```python
from build123d import *

# Parameters (mm, degrees)
SKETCH009_R     = 1.6
PAD003_DEPTH    = 2.5
SKETCH010_R     = 1.6
PAD004_DEPTH    = 2.5
FILLET002_R     = 2
SKETCH011_R     = 6.5
SKETCH011_R_2   = 1.6
PAD005_DEPTH    = 2
SKETCH012_R     = 3.2
SKETCH012_R_2   = 1.6
PAD006_DEPTH    = 4.25
FILLET003_R     = 1
POCKET006_DEPTH = 2.5


with BuildPart() as part:
    # Sketch009 → Pad003 (new body)
    with BuildSketch(Plane.XY):
        with BuildLine():
            ThreePointArc((23.646194, 14.453806), (23.646194, 23.646194), (14.453806, 23.646194))
            Line((14.453806, 23.646194), (0, 9.192388))
            Line((-14.453806, 23.646194), (0, 9.192388))
            ThreePointArc((-14.453806, 23.646194), (-23.646194, 23.646194), (-23.646194, 14.453806))
            Line((-9.192388, 0), (-23.646194, 14.453806))
            Line((-23.646194, -14.453806), (-9.192388, 0))
            ThreePointArc((-23.646194, -14.453806), (-23.646194, -23.646194), (-14.453806, -23.646194))
            Line((-14.453806, -23.646194), (0, -9.192388))
            Line((14.453806, -23.646194), (0, -9.192388))
            ThreePointArc((14.453806, -23.646194), (23.646194, -23.646194), (23.646194, -14.453806))
            Line((23.646194, -14.453806), (9.192388, 0))
            Line((23.646194, 14.453806), (9.192388, 0))
        make_face()
        with Locations((19.05, 19.05)):
            Circle(SKETCH009_R, mode=Mode.SUBTRACT)
        with Locations((-19.05, 19.05)):
            Circle(SKETCH009_R, mode=Mode.SUBTRACT)
        with Locations((-19.05, -19.05)):
            Circle(SKETCH009_R, mode=Mode.SUBTRACT)
        with Locations((19.05, -19.05)):
            Circle(SKETCH009_R, mode=Mode.SUBTRACT)
    extrude(amount=PAD003_DEPTH)

    # Sketch010 → Pad004 (join)
    with BuildSketch(Plane.XY):
        with BuildLine():
            ThreePointArc((-25, 4.8), (-29.8, 0), (-25, -4.8))
            Line((-25, -4.8), (25, -4.8))
            ThreePointArc((25, -4.8), (29.8, 0), (25, 4.8))
            Line((25, 4.8), (-25, 4.8))
        make_face()
        with Locations((-25, 0)):
            Circle(SKETCH010_R, mode=Mode.SUBTRACT)
        with Locations((25, 0)):
            Circle(SKETCH010_R, mode=Mode.SUBTRACT)
    extrude(amount=PAD004_DEPTH)

    # Fillet002
    fillet002_edges = [part.edges().sort_by_distance(p)[0] for p in [
        (13.992388, 4.8, 1.25),
        (13.992388, -4.8, 1.25),
        (0, -9.192388, 1.25),
        (-13.992388, -4.8, 1.25),
        (-13.992388, 4.8, 1.25),
        (0, 9.192388, 1.25),
    ]]
    fillet(fillet002_edges, radius=FILLET002_R)

    # Sketch011 (on Face16 of Fillet002) → Pad005 (join)
    with BuildSketch(Plane.XY.offset(2.5)):
        with Locations((-19.05, 19.05)):
            Circle(SKETCH011_R)
        with Locations((-19.05, 19.05)):
            Circle(SKETCH011_R_2, mode=Mode.SUBTRACT)
        with Locations((19.05, 19.05)):
            Circle(SKETCH011_R)
        with Locations((19.05, 19.05)):
            Circle(SKETCH011_R_2, mode=Mode.SUBTRACT)
        with Locations((19.05, -19.05)):
            Circle(SKETCH011_R)
        with Locations((19.05, -19.05)):
            Circle(SKETCH011_R_2, mode=Mode.SUBTRACT)
        with Locations((-19.05, -19.05)):
            Circle(SKETCH011_R)
        with Locations((-19.05, -19.05)):
            Circle(SKETCH011_R_2, mode=Mode.SUBTRACT)
    extrude(amount=PAD005_DEPTH)

    # Sketch012 (on Face52 of Pad005) → Pad006 (join)
    with BuildSketch(Plane.XY.offset(4.5)):
        with Locations((-19.05, 19.05)):
            Circle(SKETCH012_R)
        with Locations((-19.05, 19.05)):
            Circle(SKETCH012_R_2, mode=Mode.SUBTRACT)
        with Locations((19.05, 19.05)):
            Circle(SKETCH012_R)
        with Locations((19.05, 19.05)):
            Circle(SKETCH012_R_2, mode=Mode.SUBTRACT)
        with Locations((19.05, -19.05)):
            Circle(SKETCH012_R)
        with Locations((19.05, -19.05)):
            Circle(SKETCH012_R_2, mode=Mode.SUBTRACT)
        with Locations((-19.05, -19.05)):
            Circle(SKETCH012_R)
        with Locations((-19.05, -19.05)):
            Circle(SKETCH012_R_2, mode=Mode.SUBTRACT)
    extrude(amount=PAD006_DEPTH)

    # Fillet003
    fillet003_edges = [part.edges().sort_by_distance(p)[0] for p in [
        (15.85, -19.05, 4.5),
        (15.85, 19.05, 4.5),
        (-22.25, 19.05, 4.5),
        (-22.25, -19.05, 4.5),
    ]]
    fillet(fillet003_edges, radius=FILLET003_R)

    # Sketch013 (on Face22 of Fillet003) → Pocket006 (cut)
    with BuildSketch(Plane(origin=(0, 0, 0), x_dir=(1, 0, 0), z_dir=(0, 0, -1))):
        Polygon((-15.8, 19.05), (-17.425, 21.864583), (-20.675, 21.864583), (-22.3, 19.05), (-20.675, 16.235417), (-17.425, 16.235417), align=None)
        Polygon((22.3, 19.05), (20.675, 21.864583), (17.425, 21.864583), (15.8, 19.05), (17.425, 16.235417), (20.675, 16.235417), align=None)
        Polygon((22.3, -19.05), (20.675, -16.235417), (17.425, -16.235417), (15.8, -19.05), (17.425, -21.864583), (20.675, -21.864583), align=None)
        Polygon((-15.8, -19.05), (-17.425, -16.235417), (-20.675, -16.235417), (-22.3, -19.05), (-20.675, -21.864583), (-17.425, -21.864583), align=None)
    extrude(amount=-POCKET006_DEPTH, mode=Mode.SUBTRACT)


solid = part.part
```
Verification items for the finished model (mm, model axes). A direction names the side the tool comes from. Coordinates: 2 decimals unless noted, no trailing zeros. Loops run counter-clockwise (first coordinate to the right, second up) from the corner with the lowest first, then second, coordinate; pieces in that order, holes last. Notation, with made-up numbers: (-6, -10) -> (22, -10) arc R31 cw to (22, 17) -> close; hole circle Ø9 at (-14, -33.75). An arc over 180 degrees is marked (long way). Put each result on its own line as item: value.
1. Section check C-C, the plane z = 1.75. Give the number of separate pieces and of enclosed holes in the cut face, then the cut area to 3 significant figures.
Result set:
separate pieces: 1
enclosed holes: 6
area: 1,720 mm^2
2. Mould release check, pull along Y, two halves, no side actions. Record for faces 6 (the face through (16.601, 20.438, 1.232)), 7 (the face through (20.4, 14.8, 4.5)), 8 (the face through (-0.02, 10.02, 1.27)), 9 (the face through (20.4, -20.4, 8.75)): pulls with the +Y half, pulls with the -Y half, needs draft (parallel to the pull), parting line crosses it, or undercut.
Result set:
face 6: undercut
face 7: undercut
face 8: pulls with the +Y half
face 9: needs draft
3. Gauge pin test, flat ends, axial feed: P1, Ø1.2, axis at x = -23.5, z = 1, coming from the +Y side; P2, Ø1.7, axis at x = -19, y = 18, coming from the -Z side; P3, Ø2, axis at x = -23.5, z = 2, coming from the -Y side. Record the tip position at first contact, or that the pin passes through.
Result set:
P1: stops at y = 24.29
P2: stops at z = 2.5
P3: stops at y = -24.56
4. Thickness scan on line 1 (Y direction, x = 19, z = 4.25); line 2 (Y direction, x = -19.05, z = 7); line 3 (X direction, y = 18.5, z = 4.75). Record the ranges inside material, lowest first.
Result set:
line 1: y = -25.55 to -20.65, -17.45 to -12.55, 12.55 to 17.45, 20.65 to 25.55
line 2: y = -22.25 to -20.65, -17.45 to -15.85, 15.85 to 17.45, 20.65 to 22.25
line 3: x = -22.55 to -20.55, -17.55 to -15.55, 15.55 to 17.55, 20.55 to 22.55
5. Section check D-D, the plane x = -2.5. Record the boundary of the cut face in (y, z).
Result set:
outline: (-11.69, 0) -> (11.69, 0) -> (11.69, 2.5) -> (-11.69, 2.5) -> close
6. Tool access check on faces 1 (the face through (20.57, -11.38, 1.23)), 2 (the face through (16.601, -17.662, 1.232)), 3 (the face through (-20.48, 11.29, 1.23)), 4 (the face through (-21, -20, 8.75)), 5 (the face through (-17.7, 14.8, 4.5)). Record the directions out of +Z, -Z, +X, -X, +Y, -Y that give a thin tool (end or side, any length) a straight path to the whole face; none if there is none.
Result set:
face 1: +Z, -Z, +X
face 2: -Z
face 3: +Z, -Z, -X
face 4: +Z, +X, -X, +Y, -Y
face 5: +Z
7. Section check B-B, the plane y = 0. Record the boundary of the cut face in (x, z).
Result set:
outline: (-29.8, 0) -> (-26.6, 0) -> (-26.6, 2.5) -> (-29.8, 2.5) -> close; (-23.4, 0) -> (23.4, 0) -> (23.4, 2.5) -> (-23.4, 2.5) -> close; (26.6, 0) -> (29.8, 0) -> (29.8, 2.5) -> (26.6, 2.5) -> close
8. Section check A-A, the plane z = 7. Record the boundary of the cut face in (x, y), then the cut area to 3 significant figures.
Result set:
outline: circle Ø6.4 at (-19.05, -19.05); circle Ø6.4 at (-19.05, 19.05); circle Ø6.4 at (19.05, -19.05); circle Ø6.4 at (19.05, 19.05); hole circle Ø3.2 at (-19.05, -19.05); hole circle Ø3.2 at (-19.05, 19.05); hole circle Ø3.2 at (19.05, -19.05); hole circle Ø3.2 at (19.05, 19.05)
area: 96.5 mm^2
